The listing builds one solid part. Answer for the finished solid, in the listing's coordinates (mm). Face numbers are marked on the shaded views. A direction names the side the tool comes from. Round coordinates to 2 decimals unless told otherwise and drop trailing zeros. Write each loop counter-clockwise with the first axis right and the second up, starting at its lowest first coordinate (ties: lowest second). Pieces come first, ordered by that corner, then holes. Notation, with made-up numbers: M 46.25,-20 L 74.25,-20 A37 ccw 74.25,16 Z; hole C -20,33 d3. An arc over 180 degrees is marked long. Put each result on its own line as item: value. Start each with the question number.
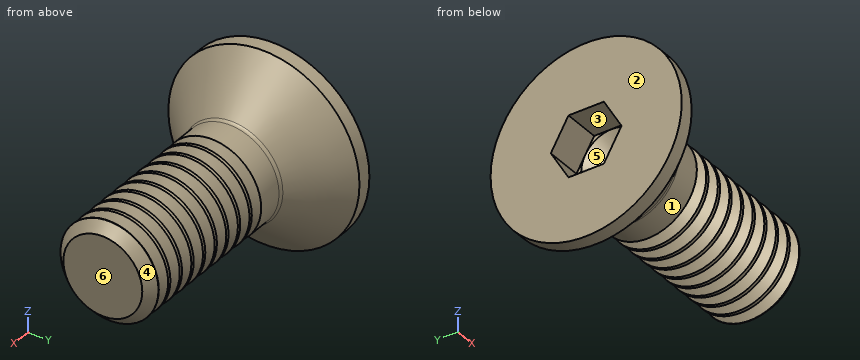
```python
from build123d import *

# Parameters (mm, degrees)
FILLET1_R       = 0.2
HEX_2_DEPTH     = 1.5
THDSCHPAT_COUNT = 9
THDSCHPAT_PITCH = 0.68


with BuildPart() as part:
    # BodySke → BaseBody (revolve)
    with BuildSketch(Plane.XY):
        Polygon((0, 0), (0, 3.9), (0.58, 3.9), (2.48, 2), (9.61, 2), (10, 1.61), (10, 0), align=None)
    revolve(axis=Axis((0, 0, 0), (1, 0, 0)))

    # Fillet1
    fillet1_edges = [part.edges().sort_by_distance(p)[0] for p in [
        (2.48, -2, 0),
    ]]
    fillet(fillet1_edges, radius=FILLET1_R)

    # Sketch2 → PreBroach (revolve, cut)
    with BuildSketch(Plane.XY):
        Polygon((0, 1.25), (1.5, 1.25), (2.221687836, 0), (0, 0), align=None)
    revolve(axis=Axis((0, 0, 0), (1, 0, 0)), mode=Mode.SUBTRACT)

    # Sketch3 → Hex 2 (cut)
    with BuildSketch(Plane.ZY):
        Polygon((-1.25, -0.721687836), (-1.25, 0.721687836), (0, 1.443375673), (1.25, 0.721687836), (1.25, -0.721687836), (0, -1.443375673), align=None)
    extrude(amount=-HEX_2_DEPTH, mode=Mode.SUBTRACT)

    # ThdSchSke → ThreadSchematic (revolve, cut)
    with BuildSketch(Plane.XY):
        Polygon((3.880001, -1.61), (3.60692006, -2), (3.60692006, -2.5), (4.15308194, -2.5), (4.15308194, -2), align=None)
    threadschematic = revolve(axis=Axis((-3.175, 0, 0), (1, 0, 0)), mode=Mode.SUBTRACT)

    # ThdSchPat: ThreadSchematic ×9
    with Locations(*[(i * THDSCHPAT_PITCH, 0, 0) for i in range(1, THDSCHPAT_COUNT)]):
        add(threadschematic, mode=Mode.SUBTRACT)


solid = part.part
```
Item 1: Which of the six approach directions +Z, -Z, +X, -X, +Y, -Y give full straight-line access (tool end or side, diameter ignored) to the marked faces 1, 2 and 3?
Item 2: Flat-ended cylindrical pins translate along their axes: pin 1 (1.2 mm diameter, centred on x = 0.5, y = 0.5, fed in from +Z); pin 2 (1 mm diameter, centred on x = 9, y = 2, fed in from -Z); pin 3 (3 mm diameter, centred on x = 7.5, y = 2, fed in from -Z). Find the tip coordinate at first contact, or state that the pin passes through.
Item 3: Consider line 1 along Y through (x, z) = (0.75, 0.25); line 2 along Y through (x, z) = (6.25, 1.75); line 3 along X through (y, z) = (-1.75, 2). Determine where each line is inside the solid, lowest interval first. Write a range as [from, to].
Item 4: Determine the mould class of the marked faces 4, 5 and 6 for opening direction Z: released by +Z, released by -Z, zero draft, split by the parting line, or undercut.
Item 5: Section A-A (x = 3.75) is taken. Give the vertices of the cut face in (y, z), and give its area (3 significant figures).
Output values:
1. face 1: +X
1. face 2: +Z, -Z, -X, +Y, -Y
1. face 3: -X
2. pin 1: stops at z = 3.9
2. pin 2: stops at z = -1.32
2. pin 3: stops at z = -1.94
3. line 1: y = [-3.72, -1.3], [1.3, 3.72]
3. line 2: y = [-0.97, 0.97]
3. line 3: x = [0, 1.82]
4. face 4: split by the parting line
4. face 5: undercut
4. face 6: zero draft
5. outline: C 0,0 d3.59
5. area: 10.1 mm^2
